Check sheet for the modelled part. Datum: model origin and axes. Units: mm. Face numbers are marked on the shaded views. Round coordinates to 2 decimals unless told otherwise and drop trailing zeros. Order: outer loops, then holes, each group sorted by start corner. A loop starts at its lowest first (then second) coordinate and runs counter-clockwise, first axis right, second up.
```python
from build123d import *

# Parameters (mm, degrees)
ESQUISSE1_W        = 100
ESQUISSE1_H        = 100
ESQUISSE1_R        = 1.5
ESQUISSE1_R_2      = 1
BOSS_EXTRU_1_DEPTH = 3
CONG_1_R           = 20
CONG_2_R           = 5
CONG_3_R           = 4
CONG_4_R           = 2


with BuildPart() as part:
    # Esquisse1 → Boss.-Extru.1 (new body)
    with BuildSketch(Plane(origin=(0, 0, 0), x_dir=(1, 0, 0), z_dir=(0, 1, 0))):
        Rectangle(ESQUISSE1_W, ESQUISSE1_H)
        with Locations((-12.5, -12.5)):
            Circle(ESQUISSE1_R, mode=Mode.SUBTRACT)
        with Locations((12.5, -12.5)):
            Circle(ESQUISSE1_R, mode=Mode.SUBTRACT)
        with Locations((-12.5, 12.5)):
            Circle(ESQUISSE1_R, mode=Mode.SUBTRACT)
        with Locations((12.5, 12.5)):
            Circle(ESQUISSE1_R, mode=Mode.SUBTRACT)
        with Locations((40.707106781, -29.393398282)):
            Circle(ESQUISSE1_R_2, mode=Mode.SUBTRACT)
        with Locations((29.393398282, -40.707106781)):
            Circle(ESQUISSE1_R_2, mode=Mode.SUBTRACT)
        with Locations((-29.393398282, -40.707106781)):
            Circle(ESQUISSE1_R_2, mode=Mode.SUBTRACT)
        with Locations((-40.707106781, -29.393398282)):
            Circle(ESQUISSE1_R_2, mode=Mode.SUBTRACT)
        with Locations((-40.707106781, 29.393398282)):
            Circle(ESQUISSE1_R_2, mode=Mode.SUBTRACT)
        with Locations((-29.393398282, 40.707106781)):
            Circle(ESQUISSE1_R_2, mode=Mode.SUBTRACT)
        with Locations((29.393398282, 40.707106781)):
            Circle(ESQUISSE1_R_2, mode=Mode.SUBTRACT)
        with Locations((40.707106781, 29.393398282)):
            Circle(ESQUISSE1_R_2, mode=Mode.SUBTRACT)
        Polygon((-9.261402822, -16), (0, -36.375086208), (9.261402822, -16), align=None, mode=Mode.SUBTRACT)
        Polygon((0, -1.414213562), (-9.585786438, -11), (9.585786438, -11), align=None, mode=Mode.SUBTRACT)
        Polygon((-34.964466094, -38.5), (-2.329506269, -38.5), (-12.527931214, -16.06346512), align=None, mode=Mode.SUBTRACT)
        Polygon((34.964466094, -38.5), (2.329506269, -38.5), (12.527931214, -16.06346512), align=None, mode=Mode.SUBTRACT)
        Polygon((-16, 9.261402822), (-36.375086208, 0), (-16, -9.261402822), align=None, mode=Mode.SUBTRACT)
        Polygon((-1.414213562, 0), (-11, 9.585786438), (-11, -9.585786438), align=None, mode=Mode.SUBTRACT)
        Polygon((-38.5, 34.964466094), (-38.5, 2.329506269), (-16.06346512, 12.527931214), align=None, mode=Mode.SUBTRACT)
        Polygon((-38.5, -34.964466094), (-38.5, -2.329506269), (-16.06346512, -12.527931214), align=None, mode=Mode.SUBTRACT)
        Polygon((9.261402822, 16), (0, 36.375086208), (-9.261402822, 16), align=None, mode=Mode.SUBTRACT)
        Polygon((0, 1.414213562), (9.585786438, 11), (-9.585786438, 11), align=None, mode=Mode.SUBTRACT)
        Polygon((34.964466094, 38.5), (2.329506269, 38.5), (12.527931214, 16.06346512), align=None, mode=Mode.SUBTRACT)
        Polygon((-34.964466094, 38.5), (-2.329506269, 38.5), (-12.527931214, 16.06346512), align=None, mode=Mode.SUBTRACT)
        Polygon((16, -9.261402822), (36.375086208, 0), (16, 9.261402822), align=None, mode=Mode.SUBTRACT)
        Polygon((1.414213562, 0), (11, -9.585786438), (11, 9.585786438), align=None, mode=Mode.SUBTRACT)
        Polygon((38.5, -34.964466094), (38.5, -2.329506269), (16.06346512, -12.527931214), align=None, mode=Mode.SUBTRACT)
        Polygon((38.5, 34.964466094), (38.5, 2.329506269), (16.06346512, 12.527931214), align=None, mode=Mode.SUBTRACT)
    extrude(amount=BOSS_EXTRU_1_DEPTH)

    # Congé1
    cong_1_edges = [part.edges().sort_by_distance(p)[0] for p in [
        (-50, 1.5, -50),
        (50, 1.5, -50),
        (50, 1.5, 50),
        (-50, 1.5, 50),
    ]]
    fillet(cong_1_edges, radius=CONG_1_R)

    # Congé2
    cong_2_edges = [part.edges().sort_by_distance(p)[0] for p in [
        (0, 1.5, -36.375086208),
        (34.964466094, 1.5, -38.5),
        (-34.964466094, 1.5, -38.5),
        (36.375086208, 1.5, 0),
        (38.5, 1.5, 34.964466094),
        (38.5, 1.5, -34.964466094),
        (0, 1.5, 36.375086208),
        (-34.964466094, 1.5, 38.5),
        (34.964466094, 1.5, 38.5),
        (-36.375086208, 1.5, 0),
        (-38.5, 1.5, -34.964466094),
        (-38.5, 1.5, 34.964466094),
    ]]
    fillet(cong_2_edges, radius=CONG_2_R)

    # Congé3
    cong_3_edges = [part.edges().sort_by_distance(p)[0] for p in [
        (12.527931214, 1.5, -16.06346512),
        (2.329506269, 1.5, -38.5),
        (-12.527931214, 1.5, -16.06346512),
        (-2.329506269, 1.5, -38.5),
        (16.06346512, 1.5, 12.527931214),
        (38.5, 1.5, 2.329506269),
        (16.06346512, 1.5, -12.527931214),
        (38.5, 1.5, -2.329506269),
        (-12.527931214, 1.5, 16.06346512),
        (-2.329506269, 1.5, 38.5),
        (12.527931214, 1.5, 16.06346512),
        (2.329506269, 1.5, 38.5),
        (-16.06346512, 1.5, -12.527931214),
        (-38.5, 1.5, -2.329506269),
        (-16.06346512, 1.5, 12.527931214),
        (-38.5, 1.5, 2.329506269),
    ]]
    fillet(cong_3_edges, radius=CONG_3_R)

    # Congé4
    cong_4_edges = [part.edges().sort_by_distance(p)[0] for p in [
        (-9.585786438, 1.5, -11),
        (0, 1.5, -1.414213562),
        (9.585786438, 1.5, -11),
        (-9.261402822, 1.5, -16),
        (9.261402822, 1.5, -16),
        (9.585786438, 1.5, 11),
        (0, 1.5, 1.414213562),
        (11, 1.5, -9.585786438),
        (1.414213562, 1.5, 0),
        (11, 1.5, 9.585786438),
        (-9.585786438, 1.5, 11),
        (16, 1.5, -9.261402822),
        (16, 1.5, 9.261402822),
        (9.261402822, 1.5, 16),
        (-9.261402822, 1.5, 16),
        (-11, 1.5, 9.585786438),
        (-1.414213562, 1.5, 0),
        (-11, 1.5, -9.585786438),
        (-16, 1.5, 9.261402822),
        (-16, 1.5, -9.261402822),
    ]]
    fillet(cong_4_edges, radius=CONG_4_R)


solid = part.part
```
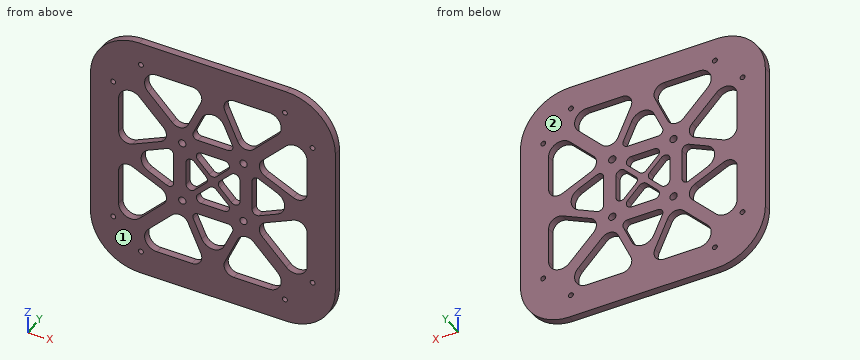
Item 1: Go/stop test with a flat-tipped pin: P1, Ø1, axis at y = 2, z = 37, coming from the -X side. Record where the tip stops, or that it passes through.
Answer:
P1: stops at x = -48.91
Item 2: Sectioned sample at A-A (z = -12.5). Record the cut outline in (x, y).
Answer:
outline: (-50, 0) - (-38.5, 0) - (-38.5, 3) - (-50, 3) - close; (-19.18, 0) - (-14, 0) - (-14, 3) - (-19.18, 3) - close; (-11, 0) - (11, 0) - (11, 3) - (-11, 3) - close; (14, 0) - (19.18, 0) - (19.18, 3) - (14, 3) - close; (38.5, 0) - (50, 0) - (50, 3) - (38.5, 3) - close
Item 3: Release check for a two-part mould opening along Y. For the marked faces 1 and 2 record: released by +Y, released by -Y, zero draft, split by the parting line, or undercut.
Answer:
face 1: released by -Y
face 2: released by +Y
Item 4: Sectioned sample at B-B (x = 12.5). Record the cut outline in (y, z), and give its area (3 significant figures).
Answer:
outline: (0, -50) - (3, -50) - (3, -38.5) - (0, -38.5) - close; (0, -19.18) - (3, -19.18) - (3, -14) - (0, -14) - close; (0, -11) - (3, -11) - (3, 11) - (0, 11) - close; (0, 14) - (3, 14) - (3, 19.18) - (0, 19.18) - close; (0, 38.5) - (3, 38.5) - (3, 50) - (0, 50) - close
area: 166 mm2
Item 5: Sectioned sample at C-C (z = -36). Record the cut outline in (x, y), and give its area (3 significant figures).
Answer:
outline: (-49.08, 0) - (-27.22, 0) - (-27.22, 3) - (-49.08, 3) - close; (-4.83, 0) - (4.83, 0) - (4.83, 3) - (-4.83, 3) - close; (27.22, 0) - (49.08, 0) - (49.08, 3) - (27.22, 3) - close
area: 160 mm2
Item 6: Sectioned sample at D-D (y = 0.8). State how many separate pieces and enclosed holes the cut face has, and give its area (3 significant figures).
Answer:
separate pieces: 1
enclosed holes: 28
area: 6,100 mm2
Item 7: Scan lines: line 1 along Z through (x, y) = (-32, 0.6); line 2 along X through (y, z) = (1.7, -16.5); line 3 along Z through (x, y) = (-12.5, 1.6). Record each from-to range of solid material in increasing order.
Answer:
line 1: z = -49.9 to -27.66, -5.28 to 5.28, 27.66 to 49.9
line 2: x = -50 to -38.5, -20.04 to -7.48, 7.48 to 20.04, 38.5 to 50
line 3: z = -50 to -38.5, -19.18 to -14, -11 to 11, 14 to 19.18, 38.5 to 50
